Could you check a few things on this model? Use its own coordinates, in mm. A direction names the side the tool comes from. Give positions to 0.01 mm unless a question says otherwise; leave off trailing zeros. Write each loop counter-clockwise with the first axis right and the second up, starting at its lowest first coordinate (ties: lowest second). Pieces come first, ordered by that corner, then holes. Notation, with made-up numbers: (6.25, 84.25) - (52.25, 84.25) arc R10 ccw to (52.25, 102.25) - close; hole circle Ø4 at (1.5, 80). An arc over 180 degrees is marked (long way). Answer in a Markdown table with one row per item.
from build123d import *

# Parameters (mm, degrees)
SKETCH_1_W           = 15.24
SKETCH_1_H           = 6.35
EXTRUDE_1_DEPTH      = 5.08
SKETCH_2_W           = 14.24
SKETCH_2_H           = 5.35
CUT_EXTRUDE_1_DEPTH  = 4.08
SKETCH_3_W           = 2
SKETCH_3_H           = 4.08
CUT_EXTRUDE_2_DEPTH  = 1
EXTRUDE_2_DEPTH      = 2
EXTRUDE_2_DEPTH_BACK = 3.58
SKETCH_4_W           = 0.75
SKETCH_4_H           = 0.75


with BuildPart() as part:
    # 草图1 → 拉伸1 (new body)
    with BuildSketch(Plane(origin=(0, 0, 0), x_dir=(1, 0, 0), z_dir=(0, 1, 0))):
        Rectangle(SKETCH_1_W, SKETCH_1_H)
    extrude(amount=EXTRUDE_1_DEPTH)

    # 草图2 → 切除-拉伸1 (cut)
    with BuildSketch(Plane(origin=(0, 5.08, 0), x_dir=(-1, 0, 0), z_dir=(0, 1, 0))):
        Rectangle(SKETCH_2_W, SKETCH_2_H)
    extrude(amount=-CUT_EXTRUDE_1_DEPTH, mode=Mode.SUBTRACT)

    # 草图3 → 切除-拉伸2 (cut)
    with BuildSketch(Plane.XY.offset(3.175)):
        with Locations((0, 3.04)):
            Rectangle(SKETCH_3_W, SKETCH_3_H)
    extrude(amount=-CUT_EXTRUDE_2_DEPTH, mode=Mode.SUBTRACT)

    # 草图4 → 拉伸2 (add, two sides: drawn at the far end of the back side and taken through both)
    with BuildSketch(Plane.XZ.offset(-EXTRUDE_2_DEPTH_BACK)):
        with Locations((-2.54, 0.635)):
            Rectangle(SKETCH_4_W, SKETCH_4_H)
        with Locations((0, 0.635)):
            Rectangle(SKETCH_4_W, SKETCH_4_H)
        with Locations((2.54, 0.635)):
            Rectangle(SKETCH_4_W, SKETCH_4_H)
        with Locations((-5.08, 0.635)):
            Rectangle(SKETCH_4_W, SKETCH_4_H)
        with Locations((5.08, 0.635)):
            Rectangle(SKETCH_4_W, SKETCH_4_H)
    extrude(amount=EXTRUDE_2_DEPTH + EXTRUDE_2_DEPTH_BACK)


solid = part.part
1) Imagine slicing it at A-A (y = 2). State how many separate pieces and enclosed holes the cut face has, then the cut area to 3 significant figures.
Check values:
| item | result |
|---|---|
| separate pieces | 6 |
| enclosed holes | 0 |
| area | 22.4 mm2 |
2) Imagine slicing it at B-B (x = -5.25). List the corners of the cut face in (y, z) for me (3 decimals).
Check values:
| item | result |
|---|---|
| outline | (-2, 0.26) - (0, 0.26) - (0, -3.175) - (5.08, -3.175) - (5.08, -2.675) - (1, -2.675) - (1, 0.26) - (3.58, 0.26) - (3.58, 1.01) - (1, 1.01) - (1, 2.675) - (5.08, 2.675) - (5.08, 3.175) - (0, 3.175) - (0, 1.01) - (-2, 1.01) - close |
3) Imagine slicing it at D-D (z = -2.25). List the corners of the cut face in (x, y) for me, then the cut area to 3 significant figures.
Check values:
| item | result |
|---|---|
| outline | (-7.62, 0) - (7.62, 0) - (7.62, 5.08) - (7.12, 5.08) - (7.12, 1) - (-7.12, 1) - (-7.12, 5.08) - (-7.62, 5.08) - close |
| area | 19.3 mm2 |
4) Will these pins go through, and if not, where does the flat tip stop? P1, Ø0.8, axis at x = -5, z = 0.5, coming from the +Y side; P2, Ø0.6, axis at y = -1, z = 0.5, coming from the -X side (3 decimals); P3, Ø1.5, axis at x = -1.5, z = -1, coming from the -Y side.
Check values:
| item | result |
|---|---|
| P1 | stops at y = 3.58 |
| P2 | stops at x = -5.455 |
| P3 | stops at y = 0 |
5) Imagine slicing it at C-C (y = -0.5). List the corners of the cut face in (x, z) for me (3 decimals).
Check values:
| item | result |
|---|---|
| outline | (-5.455, 0.26) - (-4.705, 0.26) - (-4.705, 1.01) - (-5.455, 1.01) - close; (-2.915, 0.26) - (-2.165, 0.26) - (-2.165, 1.01) - (-2.915, 1.01) - close; (-0.375, 0.26) - (0.375, 0.26) - (0.375, 1.01) - (-0.375, 1.01) - close; (2.165, 0.26) - (2.915, 0.26) - (2.915, 1.01) - (2.165, 1.01) - close; (4.705, 0.26) - (5.455, 0.26) - (5.455, 1.01) - (4.705, 1.01) - close |
6) If I drill on line 1 (Z direction, x = 5, y = 2.5) (3 decimals); line 2 (X direction, y = 3, z = 0); line 3 (Z direction, x = -3.75, y = 1.5) (3 decimals), over which ranges is the centre line in solid material (lowest first)?
Check values:
| item | result |
|---|---|
| line 1 | z = -3.175 to -2.675, 0.26 to 1.01, 2.675 to 3.175 |
| line 2 | x = -7.62 to -7.12, 7.12 to 7.62 |
| line 3 | z = -3.175 to -2.675, 2.675 to 3.175 |
7) On a 3-axis mill with a long thin cutter (end or side, diameter ignored), from which of +Z, -Z, +X, -X, +Y, -Y can I reach the whole of each face in a straight line? I mean faces 1 (the face through (-7.62, 3, 0)), 2 (the face through (7.12, 3, 0)). Say none if no direction works.
Check values:
| item | result |
|---|---|
| face 1 | +Z, -Z, -X, +Y, -Y |
| face 2 | +Y |
8) We'd pull the mould along Z, two halves only. Please class faces 3 (the face through (-0.1, 0.8, 3.175)), 4 (the face through (7.62, 3, 0)), 5 (the face through (0, 3, -2.675)), 6 (the face through (0, 3, -3.175)): +Z half, -Z half, draft (parallel to the pull), parting line (faces both ways), or undercut.
Check values:
| item | result |
|---|---|
| face 3 | +Z half |
| face 4 | draft |
| face 5 | undercut |
| face 6 | -Z half |
